Read the model definition and answer for the solid it produces. Units are mm, in the model's axes. Face numbers are marked on the shaded views. A direction names the side the tool comes from. Give positions to 0.01 mm unless a question says otherwise; leave off trailing zeros. Write each loop counter-clockwise with the first axis right and the second up, starting at its lowest first coordinate (ties: lowest second). Pieces come first, ordered by that corner, then holes. Notation, with made-up numbers: M 62,29.25 L 116,29.25 A35 ccw 116,68.25 Z; hole C -4,69.25 d7. An arc over 180 degrees is marked long. Put each result on its own line as item: value.
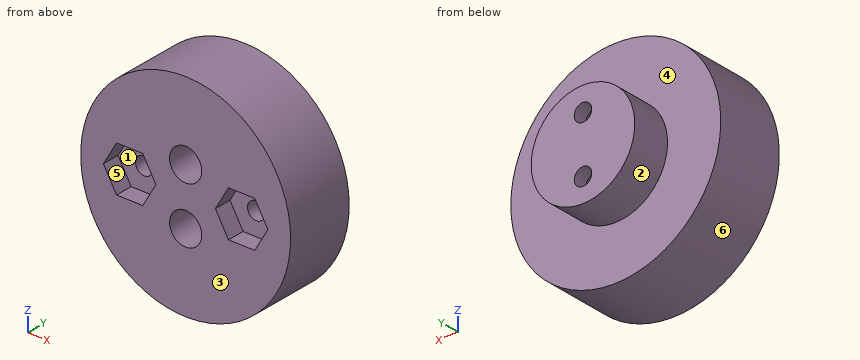
from build123d import *

# Parameters (mm, degrees)
SKETCH1_R           = 19.05
BOSS_EXTRUDE1_DEPTH = 12.7
SKETCH2_R           = 9.398
BOSS_EXTRUDE2_DEPTH = 7.112
CUT_EXTRUDE3_DEPTH  = 3.175
SKETCH6_R           = 1.5875
CUT_EXTRUDE4_DEPTH  = 7.62
SKETCH7_R           = 2.921
CUT_EXTRUDE5_DEPTH  = 17.272
SKETCH8_R           = 1.5875
CUT_EXTRUDE6_DEPTH  = 3.54


with BuildPart() as part:
    # Sketch1 → Boss-Extrude1 (new body)
    with BuildSketch(Plane(origin=(0, 0, 0), x_dir=(1, 0, 0), z_dir=(0, 1, 0))):
        Circle(SKETCH1_R)
    extrude(amount=BOSS_EXTRUDE1_DEPTH)

    # Sketch2 → Boss-Extrude2 (add)
    with BuildSketch(Plane(origin=(0, 12.7, 0), x_dir=(1, 0, 0), z_dir=(0, 1, 0))):
        Circle(SKETCH2_R)
    extrude(amount=BOSS_EXTRUDE2_DEPTH)

    # Sketch5 → Cut-Extrude3 (cut)
    with BuildSketch(Plane.XZ):
        Polygon((-5.393973528, 0), (-7.776986764, 4.1275), (-12.543013236, 4.1275), (-14.926026472, 0), (-12.543013236, -4.1275), (-7.776986764, -4.1275), align=None)
        Polygon((14.926026472, 0), (12.543013236, 4.1275), (7.776986764, 4.1275), (5.393973528, 0), (7.776986764, -4.1275), (12.543013236, -4.1275), align=None)
    extrude(amount=-CUT_EXTRUDE3_DEPTH, mode=Mode.SUBTRACT)

    # Sketch6 → Cut-Extrude4 (cut)
    with BuildSketch(Plane.XZ):
        with Locations((-10.16, 0)):
            Circle(SKETCH6_R)
        with Locations((10.16, 0)):
            Circle(SKETCH6_R)
    extrude(amount=-CUT_EXTRUDE4_DEPTH, mode=Mode.SUBTRACT)

    # Sketch7 → Cut-Extrude5 (cut)
    with BuildSketch(Plane.XZ):
        with Locations((0, 5.08)):
            Circle(SKETCH7_R)
        with Locations((0, -5.08)):
            Circle(SKETCH7_R)
    extrude(amount=-CUT_EXTRUDE5_DEPTH, mode=Mode.SUBTRACT)

    # Sketch8 → Cut-Extrude6 (cut, through all)
    with BuildSketch(Plane.XZ.offset(-17.272)):
        with Locations((0, 5.08)):
            Circle(SKETCH8_R)
        with Locations((0, -5.08)):
            Circle(SKETCH8_R)
    extrude(amount=-CUT_EXTRUDE6_DEPTH, mode=Mode.SUBTRACT)


solid = part.part
(1) Section B-B on y = 6.5 is taken. Give the number of separate pieces and of enclosed holes in the cut face, and give its area (3 significant figures).
Result:
separate pieces: 1
enclosed holes: 4
area: 1,070 mm²
(2) Section D-D on x = 10.16 is taken. Determine the outline of the cut face in (y, z) (1 decimal), and give its area (3 significant figures).
Result:
outline: M 0,-16.1 L 12.7,-16.1 L 12.7,16.1 L 0,16.1 L 0,4.1 L 3.2,4.1 L 3.2,1.6 L 7.6,1.6 L 7.6,-1.6 L 3.2,-1.6 L 3.2,-4.1 L 0,-4.1 Z
area: 369 mm²
(3) Section A-A on x = 0 is taken. Determine the outline of the cut face in (y, z).
Result:
outline: M 0,-19.05 L 12.7,-19.05 L 12.7,-9.4 L 19.81,-9.4 L 19.81,-6.67 L 17.27,-6.67 L 17.27,-8 L 0,-8 Z; M 0,-2.16 L 17.27,-2.16 L 17.27,-3.49 L 19.81,-3.49 L 19.81,3.49 L 17.27,3.49 L 17.27,2.16 L 0,2.16 Z; M 0,8 L 17.27,8 L 17.27,6.67 L 19.81,6.67 L 19.81,9.4 L 12.7,9.4 L 12.7,19.05 L 0,19.05 Z
(4) For a pull along X with two mould halves and no side action, classify the marked faces 4, 5 and 6 as +X half, -X half, draft (parallel to the pull), parting line (faces both ways), or undercut.
Result:
face 4: draft
face 5: undercut
face 6: parting line
(5) Straight lines are drawn through the part: line 1 along Z through (x, y) = (0, 9.25); line 2 along Z through (x, y) = (0, 19.05); line 3 along Y through (x, z) = (-4, -13). For each, find the intervals that lie inside material, in ascending order. Write a range as from..to.
Result:
line 1: z = -19.05..-8, -2.16..2.16, 8..19.05
line 2: z = -9.4..-6.67, -3.49..3.49, 6.67..9.4
line 3: y = 0..12.7
(6) Which of the six approach directions +Z, -Z, +X, -X, +Y, -Y give full straight-line access (tool end or side, diameter ignored) to the marked faces 1, 2 and 3?
Result:
face 1: -Y
face 2: +Y
face 3: +Z, -Z, +X, -X, -Y
(7) Given pin 1 Ø8 at (y, z) = (4, 13.5) entering from -X; pin 2 Ø12 at (x, z) = (-14, 7.5) entering from +Y; pin 3 Ø1.6 at (x, y) = (-10, 1.5) entering from +Z; pin 4 Ø1.9 at (x, z) = (0, 5.08) entering from -Y, each flat-ended and moving along its own axis, determine where each tip first touches the part or whether it passes through.
Result:
pin 1: stops at x = -16.51
pin 2: stops at y = 12.7
pin 3: stops at z = 16.68
pin 4: passes through
(8) Section C-C on z = 5.08 is taken. Determine the outline of the cut face in (x, y), and give its area (3 significant figures).
Result:
outline: M -18.36,0 L -2.92,0 L -2.92,17.27 L -1.59,17.27 L -1.59,19.81 L -7.91,19.81 L -7.91,12.7 L -18.36,12.7 Z; M 1.59,17.27 L 2.92,17.27 L 2.92,0 L 18.36,0 L 18.36,12.7 L 7.91,12.7 L 7.91,19.81 L 1.59,19.81 Z
area: 470 mm²
